Design review of the part built by this model. Coordinates are the model's own, in mm. A direction names the side the tool comes from. Coordinates: 2 decimals unless noted, no trailing zeros. Write each loop counter-clockwise with the first axis right and the second up, starting at its lowest first coordinate (ties: lowest second). Pieces come first, ordered by that corner, then holes. Notation, with made-up numbers: M 58,12 L 116,12 A24 ccw 116,35 Z; hole C 57,46.5 d1. An arc over 180 degrees is marked long. Write item = value, one per line.
```python
from build123d import *
from build123d.topology import SkipClean

# Parameters (mm, degrees)
SKETCH1_W                = 60
SKETCH1_H                = 60
BOSS_EXTRUDE1_DEPTH      = 500
BOSS_EXTRUDE6_DEPTH      = 2.5
BOSS_EXTRUDE6_DEPTH_BACK = 30
SKETCH2_R                = 12.5
CUT_EXTRUDE1_DEPTH       = 505.479930225
BOSS_EXTRUDE7_DEPTH      = 35
SKETCH7_W                = 30
SKETCH7_H                = 25
CUT_EXTRUDE2_DEPTH       = 15
SKETCH8_R                = 12.5
CUT_EXTRUDE3_DEPTH       = 22.5
SKETCH10_R               = 5
CUT_EXTRUDE4_DEPTH       = 20


with BuildPart() as part:
    # Sketch1 → Boss-Extrude1 (new body)
    with BuildSketch(Plane(origin=(0, 0, 0), x_dir=(1, 0, 0), z_dir=(0, 1, 0))):
        Rectangle(SKETCH1_W, SKETCH1_H)
    extrude(amount=BOSS_EXTRUDE1_DEPTH)

    # Sketch2 → Boss-Extrude6 (add, two sides: drawn at the far end of the back side and taken through both)
    with BuildSketch(Plane(origin=(30, 0, 0), x_dir=(0, 0, -1), z_dir=(1, 0, 0)).offset(-BOSS_EXTRUDE6_DEPTH_BACK)):
        Circle(SKETCH2_R)
    extrude(amount=BOSS_EXTRUDE6_DEPTH + BOSS_EXTRUDE6_DEPTH_BACK)

    # Sketch5 → Cut-Extrude1 (cut, through all)
    with SkipClean():  # the faces are left unmerged after this step: merging them gives an invalid solid
        with BuildSketch(Plane(origin=(30, 0, 0), x_dir=(0, 0, -1), z_dir=(1, 0, 0))):
            with BuildLine():
                Line((-30, 0), (-30, 80))
                Line((-30, 80), (30, 80))
                Line((30, 80), (30, 0))
                Line((30, 0), (12.5, 0))
                ThreePointArc((12.5, 0), (0, 12.5), (-12.5, 0))
                Line((-12.5, 0), (-30, 0))
            make_face()
        extrude(amount=-CUT_EXTRUDE1_DEPTH, mode=Mode.SUBTRACT)


with BuildPart() as cut_extrude1_piece_1:
    # of the separate pieces the step leaves, piece 1, a body of its own (cut_extrude1_pieces)
    add(part.part.solids().sort_by_distance((30, 80, -30))[0])



with BuildPart() as cut_extrude1_piece_2:
    # of the separate pieces the step leaves, piece 2, a body of its own (cut_extrude1_pieces)
    add(part.part.solids().sort_by_distance((0, 0, 12.5))[0])


with BuildPart() as cut_extrude1_piece_1_1:
    add(cut_extrude1_piece_1.part)

    add(cut_extrude1_piece_2.part)  # Boss-Extrude7 merges Cut-Extrude1 piece 2
    # Sketch6 → Boss-Extrude7 (add)
    with BuildSketch(Plane(origin=(30, 0, 0), x_dir=(0, 0, -1), z_dir=(1, 0, 0))):
        with BuildLine():
            Line((35.819788787, 110), (35.819788787, 0))
            ThreePointArc((35.819788787, 0), (0, -35.819788787), (-35.819788787, 0))
            Line((-35.819788787, 0), (-35.819788787, 110))
            ThreePointArc((-35.819788787, 110), (0, 145.819788787), (35.819788787, 110))
        make_face()
    extrude(amount=BOSS_EXTRUDE7_DEPTH)

    # Sketch7 → Cut-Extrude2 (cut)
    with BuildSketch(Plane.XZ):
        with Locations((-15, 0)):
            Rectangle(SKETCH7_W, SKETCH7_H)
    extrude(amount=-CUT_EXTRUDE2_DEPTH, mode=Mode.SUBTRACT)

    # Sketch8 → Cut-Extrude3 (cut)
    with BuildSketch(Plane.ZY):
        with Locations(Location((0, 0, 0), (0, 0, 180))):
            Circle(SKETCH8_R)
    extrude(amount=-CUT_EXTRUDE3_DEPTH, mode=Mode.SUBTRACT)

    # Sketch10 → Cut-Extrude4 (cut)
    with BuildSketch(Plane(origin=(0, 500, 0), x_dir=(1, 0, 0), z_dir=(0, 1, 0))):
        with Locations(Location((0, 0, 0), (0, 0, 270))):
            Circle(SKETCH10_R)
    extrude(amount=-CUT_EXTRUDE4_DEPTH, mode=Mode.SUBTRACT)


solid = cut_extrude1_piece_1_1.part
```
Q1. Consider section B-B, the plane x = 0. State the section outline as (y, z) points, and give its area (3 significant figures).
Check result:
outline = M 80,-30 L 500,-30 L 500,-5 L 480,-5 L 480,5 L 500,5 L 500,30 L 80,30 Z
area = 25,000 mm²
Q2. Consider section D-D, the plane x = 56. State the section outline as (y, z) points.
Check result:
outline = M 0,-35.82 L 110,-35.82 A35.82 ccw 110,35.82 L 0,35.82 A35.82 ccw Z
Q3. The part is to be moulded in two halves that separate along Z. For faces 4 (the cylindrical face through (-4.88, 490.14, -1.08)), 5 (the flat face through (47, 56, -35.82)), 6 (the flat face through (0, 80, 0)), 7 (the flat face through (0, 480, 0)), say which applies: +Z half, -Z half, draft (parallel to the pull), parting line (faces both ways), or undercut.
Check result:
face_4 = undercut
face_5 = -Z half
face_6 = draft
face_7 = undercut
Q4. Machinability: for faces 1 (the cylindrical face through (47.26, 145.81, 0.79)), 2 (the flat face through (22.5, 0, 0)), 3 (the cylindrical face through (26.197, 3.755, -11.923)), which of the approach directions +Z, -Z, +X, -X, +Y, -Y give a long, thin tool a straight path to every point of the face, cutting with its end or side? Answer none if there is none.
Check result:
face_1 = +X, +Y
face_2 = +Z, -Z, -X, -Y
face_3 = -X
Q5. Consider section C-C, the plane y = 302. State the section outline as (x, z) points, and give its area (3 significant figures).
Check result:
outline = M -30,-30 L 30,-30 L 30,30 L -30,30 Z
area = 3,600 mm²
Q6. Wall thickness on line 1 (X direction, y = 484, z = 0); line 2 (Y direction, x = 10.5, z = -6); line 3 (Z direction, x = -20.5, y = 257.5): over which ranges is each line inside the solid? List them lowest first.
Check result:
line_1 = -30 to -5, 5 to 30
line_2 = 80 to 500
line_3 = -30 to 30
Q7. For P1, Ø3, axis at y = 391, z = 15, coming from the +X side; P2, Ø5, axis at x = -0.5, z = -2, coming from the +Y side; P3, Ø1, axis at x = -3.5, y = 345.5, coming from the +Z side, all flat-tipped, find the tip position at first contact; note any pin that passes through.
Check result:
P1 = 30
P2 = 480
P3 = 30
Q8. Consider section A-A, the plane z = 0. State the section outline as (x, y) points.
Check result:
outline = M -30,80 L 30,80 L 30,12.5 L 22.5,12.5 L 22.5,-12.5 L 30,-12.5 L 30,-35.82 L 65,-35.82 L 65,145.82 L 30,145.82 L 30,500 L 5,500 L 5,480 L -5,480 L -5,500 L -30,500 Z
